Read the model definition and answer for the solid it produces. Units are mm, in the model's axes. Face numbers are marked on the shaded views. A direction names the side the tool comes from. Coordinates: 2 decimals unless noted, no trailing zeros. Loops run counter-clockwise (first coordinate to the right, second up) from the corner with the lowest first, then second, coordinate; pieces in that order, holes last. Notation, with made-up numbers: M -40,73 L -10,73 A15 ccw -10,88 Z; hole C 78,-15.5 d10. An arc over 180 degrees is marked long. Use one line per item in the form item = value. Start each with the question number.
1. The part is cut by section A-A (y = 0). Give the vertices of the cut face in (x, z), plus the area to 3 significant figures.
2. Find the intervals of material crossed by probe 1 along X at (y, z) = (-0.25, 1.75); probe 2 along Y at (x, z) = (0, 0.45); probe 3 along Y at (x, z) = (-2, 3.8), in increasing order. Write a range as [from, to].
3. For a pull along X with two mould halves and no side action, classify the marked faces 4, 5, 6 and 7 as released by +X, released by -X, zero draft, split by the parting line, or undercut.
4. The part is cut by section D-D (y = -4.75). Give the vertices of the cut face in (x, z).
5. The part is cut by section C-C (z = 0.8). Give the vertices of the cut face in (x, y), plus the area to 3 significant figures.
6. Flat-ended cylindrical pins translate along their axes: pin 1 (3 mm diameter, centred on y = -2, z = 4.5, fed in from -X); pin 2 (0.8 mm diameter, centred on x = -4.5, y = 2.5, fed in from -Z); pin 3 (4 mm diameter, centred on x = 0, y = 0, fed in from +Z); pin 4 (1.2 mm diameter, centred on y = 3.5, z = 0.5, fed in from -X). Find the tip coordinate at first contact, or state that the pin passes through.
7. The part is cut by section B-B (x = 1). Give the vertices of the cut face in (y, z), plus the area to 3 significant figures.
8. A tool of negligible diameter and unlimited length cuts with its end or side. For the marked faces 1, 2 and 3, from which of +Z, -Z, +X, -X, +Y, -Y can it reach the whole face along a straight path? Write none if from no direction.
from build123d import *

# Parameters (mm, degrees)
BOSS_EXTRUDE1_DEPTH = 7.5
SKETCH2_R           = 2.25
CUT_EXTRUDE1_DEPTH  = 11.559356041
CUT_EXTRUDE2_START  = -3.3
CUT_EXTRUDE2_DEPTH  = 14.859356041
CUT_EXTRUDE2_DRAFT  = -2


with BuildPart() as part:
    # Sketch1 → Boss-Extrude1 (new, symmetric)
    with BuildSketch(Plane(origin=(0, 0, 0), x_dir=(1, 0, 0), z_dir=(0, 1, 0))):
        Polygon((-2.95, 0), (2.95, 0), (2.95, -1.5), (5.5, -1.5), (5.5, -2.5), (2.5, -5), (-2.5, -5), (-5.5, -2.5), (-5.5, -1.5), (-2.95, -1.5), align=None)
    extrude(amount=BOSS_EXTRUDE1_DEPTH, both=True)

    # Sketch2 → Cut-Extrude1 (cut, through all)
    with BuildSketch(Plane.XY.offset(5)):
        Circle(SKETCH2_R)
    extrude(amount=-CUT_EXTRUDE1_DEPTH, mode=Mode.SUBTRACT)


with BuildPart() as cut_extrude2_tool:
    # Sketch3 → Cut-Extrude2 (with draft: the straight prism first)
    with BuildSketch(Plane.XY.offset(5).offset(CUT_EXTRUDE2_START)):
        Polygon((0, 4.214656965), (-3.65, 2.107328483), (-3.65, -2.107328483), (0, -4.214656965), (3.65, -2.107328483), (3.65, 2.107328483), align=None)
    extrude(amount=CUT_EXTRUDE2_DEPTH)
    # Cut-Extrude2: the draft: its side faces are tilted about the plane it starts from
    cut_extrude2_sides = [cut_extrude2_tool.faces().sort_by_distance(p)[0] for p in [
        (-1.825, 3.160992724, 9.12967802),
        (-3.65, 0, 9.12967802),
        (-1.825, -3.160992724, 9.12967802),
        (1.825, -3.160992724, 9.12967802),
        (3.65, 0, 9.12967802),
        (1.825, 3.160992724, 9.12967802),
    ]]
    draft(cut_extrude2_sides, Plane.XY.offset(5).offset(CUT_EXTRUDE2_START), CUT_EXTRUDE2_DRAFT)


with BuildPart() as part_1:
    add(part.part)

    # Cut-Extrude2: cut by cut_extrude2_tool
    add(cut_extrude2_tool.part, mode=Mode.SUBTRACT)


solid = part_1.part
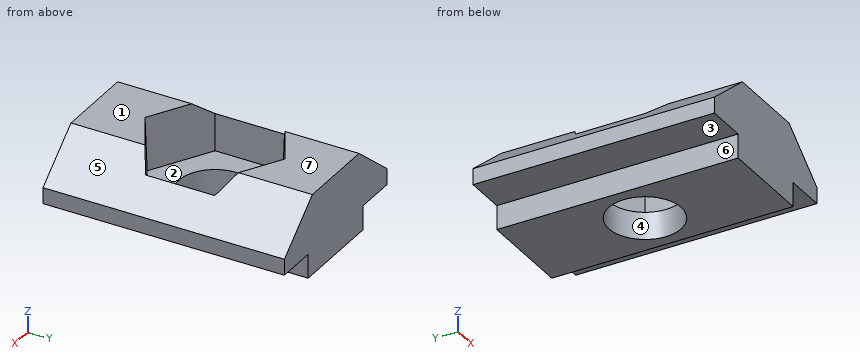
Computed values:
q1.outline = M -5.5,1.5 L -2.95,1.5 L -2.95,0 L -2.25,0 L -2.25,1.7 L -3.65,1.7 L -3.73,3.98 L -5.5,2.5 Z; M 2.25,0 L 2.95,0 L 2.95,1.5 L 5.5,1.5 L 5.5,2.5 L 3.73,3.98 L 3.65,1.7 L 2.25,1.7 Z
q1.area = 9.03 mm²
q2.probe_1 = [-5.5, -3.65], [3.65, 5.5]
q2.probe_2 = [-7.5, -2.25], [2.25, 7.5]
q2.probe_3 = [-7.5, -3.14], [3.14, 7.5]
q3.face_4 = undercut
q3.face_5 = released by +X
q3.face_6 = released by -X
q3.face_7 = zero draft
q4.outline = M -5.5,1.5 L -2.95,1.5 L -2.95,0 L 2.95,0 L 2.95,1.5 L 5.5,1.5 L 5.5,2.5 L 2.5,5 L -2.5,5 L -5.5,2.5 Z
q5.outline = M -2.95,-7.5 L 2.95,-7.5 L 2.95,7.5 L -2.95,7.5 Z; hole C 0,0 d4.5
q5.area = 72.6 mm²
q6.pin_1 = -4.9
q6.pin_2 = 1.5
q6.pin_3 = through
q6.pin_4 = -2.95
q7.outline = M -7.5,0 L -2.02,0 L -2.02,1.7 L -3.64,1.7 L -3.77,5 L -7.5,5 Z; M 2.02,0 L 7.5,0 L 7.5,5 L 3.77,5 L 3.64,1.7 L 2.02,1.7 Z
q7.area = 43.7 mm²
q8.face_1 = +Z, +X, -X, +Y, -Y
q8.face_2 = +Z
q8.face_3 = -Z, -X, +Y, -Y
